```python
from build123d import *

# Parameters (mm, degrees)
F1_DEPTH = 165.1
F2_DEPTH = 127
F4_DEPTH = 146.05


# Not quite as in the source:
# - a feature names something its author has since deleted; it is built from what else it names


with BuildPart() as f1:
    # F0 (on Front) → F1 (new body)
    with BuildSketch(Plane.XZ):
        Polygon((-0.2583676879, 64.8191452859), (-56.2642103132, 32.1858196618), (-56.0058426253, -32.6333256242), (0.2583676879, -64.8191452859), (56.2642103132, -32.1858196618), (56.0058426253, 32.6333256242), align=None)
    extrude(amount=F1_DEPTH)

    # F0 (on Front) → F2 (join)
    with BuildSketch(Plane.XZ):
        Polygon((-0.2583676879, 64.8191452859), (-56.2642103132, 32.1858196618), (-56.0058426253, -32.6333256242), (0.2583676879, -64.8191452859), (56.2642103132, -32.1858196618), (56.0058426253, 32.6333256242), align=None)
    extrude(amount=F2_DEPTH)

    # F3 (on face) → F4 (cut)
    with BuildSketch(Plane.XZ.offset(165.1)):
        Polygon((-0.1502408993, 58.3915630752), (-50.6436974394, 29.0656691021), (-50.4934565401, -29.3258939731), (0.1502408993, -58.3915630752), (50.6436974394, -29.0656691021), (50.4934565401, 29.3258939731), align=None)
    extrude(amount=-F4_DEPTH, mode=Mode.SUBTRACT)


solid = f1.part
```
Verification items for the finished model (mm, model axes). A direction names the side the tool comes from. Coordinates: 2 decimals unless noted, no trailing zeros. Order: outer loops, then holes, each group sorted by start corner. A loop starts at its lowest first (then second) coordinate and runs counter-clockwise, first axis right, second up. Notation, with made-up numbers: (77, 21.25) -> (100, 21.25) arc R21 ccw to (100, 32.25) -> close; hole circle Ø3 at (82, 18). An arc over 180 degrees is marked (long way). Put each result on its own line as item: value. Start each with the question number.
1) Material ranges on L1, parallel to X at y = -58, z = 28; L2, parallel to Y at x = 3.5, z = 44.5; L3, parallel to X at y = -82, z = 55, recorded low to high.
2) Cross-section at A-A (y = -33.5). Enter the section's corners in (x, z), plus the area to 3 significant figures.
3) Cross-section at C-C (z = -45.5). Enter the section's corners in (x, y), plus the area to 3 significant figures.
4) Tool access check on faces 4 (the flat face through (-1, 0, 1)), 5 (the flat face through (-25.044, -93.097, 43.934)). Record the directions out of +Z, -Z, +X, -X, +Y, -Y that give a thin tool (end or side, any length) a straight path to the whole face; none if there is none.
5) Release check for a two-part mould opening along Z. For faces 1 (the flat face through (-27.87, -81.39, 48.73)), 2 (the flat face through (21, -165.1, -48)), 3 (the flat face through (-1, -19.05, 1)) record: pulls with the +Z half, pulls with the -Z half, needs draft (parallel to the pull), parting line crosses it, or undercut.
6) Cross-section at B-B (x = -24.5). Enter the section's corners in (y, z), plus the area to 3 significant figures.
7) Go/stop test with flat-tipped pins: pin 1 (1 mm diameter, centred on y = -34.5, z = 47, fed in from +X); pin 2 (1.5 mm diameter, centred on x = 5.5, z = -2, fed in from -Y); pin 3 (1.5 mm diameter, centred on x = 44.5, y = -91, fed in from -Z). Record where each tip stops, or that it passes through.
8) Cross-section at D-D (y = -12). Enter the section's corners in (x, z), plus the area to 3 significant figures.
Geometry check:
1. L1: x = -56.25 to -50.64, 50.5 to 56.02
1. L2: y = -19.05 to 0
1. L3: x = -17.11 to -5.99, 5.76 to 16.91
2. outline: (-56.26, 32.19) -> (-56.01, -32.63) -> (0.26, -64.82) -> (56.26, -32.19) -> (56.01, 32.63) -> (-0.26, 64.82) -> close; hole (-50.64, 29.07) -> (-50.49, -29.33) -> (0.15, -58.39) -> (50.64, -29.07) -> (50.49, 29.33) -> (-0.15, 58.39) -> close
2. area: 2,060 mm^2
3. outline: (-33.51, -165.1) -> (-22.31, -165.1) -> (-22.31, -19.05) -> (22.35, -19.05) -> (22.35, -165.1) -> (33.41, -165.1) -> (33.41, 0) -> (-33.51, 0) -> close
3. area: 4,530 mm^2
4. face 4: +Z, -Z, +X, -X, +Y
4. face 5: -Y
5. face 1: pulls with the +Z half
5. face 2: needs draft
5. face 3: undercut
6. outline: (-165.1, -50.66) -> (0, -50.66) -> (0, 50.69) -> (-165.1, 50.69) -> (-165.1, 44.25) -> (-19.05, 44.25) -> (-19.05, -44.24) -> (-165.1, -44.24) -> close
6. area: 3,810 mm^2
7. pin 1: stops at x = 31.77
7. pin 2: stops at y = -19.05
7. pin 3: stops at z = -39.48
8. outline: (-56.26, 32.19) -> (-56.01, -32.63) -> (0.26, -64.82) -> (56.26, -32.19) -> (56.01, 32.63) -> (-0.26, 64.82) -> close
8. area: 10,900 mm^2
